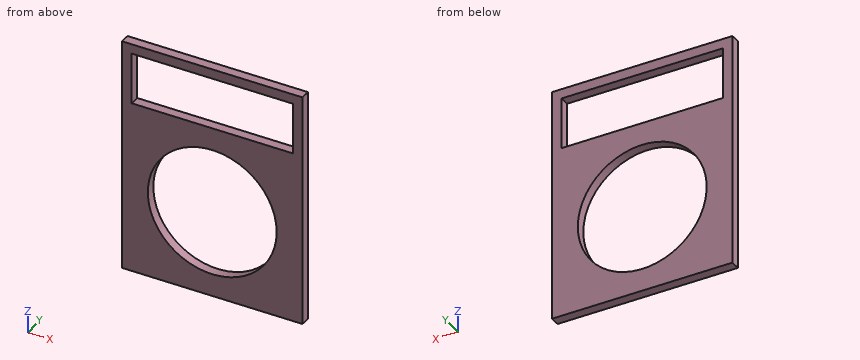
```python
from build123d import *

# Parameters (mm, degrees)
F0_W     = 355.6
F0_H     = 463.55
F1_DEPTH = 19.05
F2_W     = 317.5
F2_H     = 101.6
F3_DEPTH = 19.051
F4_R     = 127
F5_DEPTH = 19.051


with BuildPart() as f1:
    # F0 (on Front) → F1 (new body)
    with BuildSketch(Plane.XZ):
        Rectangle(F0_W, F0_H)
    extrude(amount=F1_DEPTH)

    # F2 (on face) → F3 (cut, through all)
    with BuildSketch(Plane.XZ.offset(19.05)):
        with Locations((0, 161.925)):
            Rectangle(F2_W, F2_H)
    extrude(amount=-F3_DEPTH, mode=Mode.SUBTRACT)

    # F4 (on face) → F5 (cut, through all)
    with BuildSketch(Plane.XZ.offset(19.05)):
        with Locations((0, -60.325)):
            Circle(F4_R)
    extrude(amount=-F5_DEPTH, mode=Mode.SUBTRACT)


solid = f1.part
```
Geometry: final body of the model. Coordinates: model frame, mm. Coordinates: 2 decimals unless noted, no trailing zeros. Write each loop counter-clockwise with the first axis right and the second up, starting at its lowest first coordinate (ties: lowest second). Pieces come first, ordered by that corner, then holes. Notation, with made-up numbers: M 60,63 L 94,63 A17 cw 94,94 Z; hole C 74,62.5 d8. An arc over 180 degrees is marked long. Answer as CSV lines item,"result". Start each with the question number.
Q1. Cut plane B-B on z = -76.5. Return the cut outline in (x, y).
Q2. Line query: line 1 (Z direction, x = 0, y = -4.75) (3 decimals); line 2 (Z direction, x = -5, y = -1.5) (3 decimals); line 3 (X direction, y = -5.75, z = 185.5). Output: solid intervals per line, ascending. Write a range as from..to.
Q3. Pin query (flat end, axial travel): P1, Ø10, axis at x = -117, z = -109, coming from the +Y side. Return the tip coordinate at first contact, or that it passes through.
Q4. Cut plane A-A on x = 0. Return the cut outline in (y, z) (3 decimals).
Q5. Cut plane C-C on y = -15. Return the cut outline in (x, z) (3 decimals).
Q6. Cut plane D-D on x = 91.5. Return the cut outline in (y, z) (3 decimals).
Findings below:
1,outline,"M -177.8,-19.05 L -125.97,-19.05 L -125.97,0 L -177.8,0 Z; M 125.97,-19.05 L 177.8,-19.05 L 177.8,0 L 125.97,0 Z"
2,line 1,"z = -231.775..-187.325, 66.675..111.125, 212.725..231.775"
2,line 2,"z = -231.775..-187.227, 66.577..111.125, 212.725..231.775"
2,line 3,"x = -177.8..-158.75, 158.75..177.8"
3,P1,"stops at y = 0"
4,outline,"M -19.05,-231.775 L 0,-231.775 L 0,-187.325 L -19.05,-187.325 Z; M -19.05,66.675 L 0,66.675 L 0,111.125 L -19.05,111.125 Z; M -19.05,212.725 L 0,212.725 L 0,231.775 L -19.05,231.775 Z"
5,outline,"M -177.8,-231.775 L 177.8,-231.775 L 177.8,231.775 L -177.8,231.775 Z; hole M -158.75,111.125 L 158.75,111.125 L 158.75,212.725 L -158.75,212.725 Z; hole C 0,-60.325 d254"
6,outline,"M -19.05,-231.775 L 0,-231.775 L 0,-148.397 L -19.05,-148.397 Z; M -19.05,27.747 L 0,27.747 L 0,111.125 L -19.05,111.125 Z; M -19.05,212.725 L 0,212.725 L 0,231.775 L -19.05,231.775 Z"
